from build123d import *

# Parameters (mm, degrees)
SKETCH1_W           = 19.05
SKETCH1_H           = 25.4
BOSS_EXTRUDE1_DEPTH = 6.35
SKETCH2_W           = 6.35
SKETCH2_H           = 6.35
CUT_EXTRUDE1_DEPTH  = 7.35
SKETCH3_W           = 6.35
SKETCH3_H           = 6.35
CUT_EXTRUDE2_DEPTH  = 7.35
SKETCH4_R           = 0.635
CUT_EXTRUDE3_DEPTH  = 7.35
SKETCH5_R           = 0.635
CUT_EXTRUDE4_DEPTH  = 7.35


with BuildPart() as part:
    # Sketch1 → Boss-Extrude1 (new body)
    with BuildSketch(Plane.XY):
        with Locations((9.525, 12.7)):
            Rectangle(SKETCH1_W, SKETCH1_H)
    extrude(amount=BOSS_EXTRUDE1_DEPTH)

    # Sketch2 → Cut-Extrude1 (cut, through all)
    with BuildSketch(Plane(origin=(0, 0, 0), x_dir=(-1, 0, 0), z_dir=(0, 0, -1))):
        with Locations((-3.175, 22.225)):
            Rectangle(SKETCH2_W, SKETCH2_H)
    extrude(amount=-CUT_EXTRUDE1_DEPTH, mode=Mode.SUBTRACT)

    # Sketch3 → Cut-Extrude2 (cut, through all)
    with BuildSketch(Plane(origin=(0, 0, 0), x_dir=(-1, 0, 0), z_dir=(0, 0, -1))):
        with Locations((-15.875, 22.225)):
            Rectangle(SKETCH3_W, SKETCH3_H)
    extrude(amount=-CUT_EXTRUDE2_DEPTH, mode=Mode.SUBTRACT)

    # Sketch4 → Cut-Extrude3 (cut, through all)
    with BuildSketch(Plane(origin=(0, 0, 0), x_dir=(-1, 0, 0), z_dir=(0, 0, -1))):
        with Locations((-9.525, 22.225)):
            Circle(SKETCH4_R)
    extrude(amount=-CUT_EXTRUDE3_DEPTH, mode=Mode.SUBTRACT)

    # Sketch5 → Cut-Extrude4 (cut, through all)
    with BuildSketch(Plane.XY.offset(6.35)):
        with Locations((14.2875, 3.922050028)):
            Circle(SKETCH5_R)
        with Locations((9.525, 3.922050028)):
            Circle(SKETCH5_R)
        with Locations((4.7625, 3.922050028)):
            Circle(SKETCH5_R)
    extrude(amount=-CUT_EXTRUDE4_DEPTH, mode=Mode.SUBTRACT)


solid = part.part
Source: CAD feature listing. Evaluate the final solid. Frame: model axes, mm. A direction names the side the tool comes from. Round coordinates to 2 decimals unless told otherwise and drop trailing zeros. Order: outer loops, then holes, each group sorted by start corner. A loop starts at its lowest first (then second) coordinate and runs counter-clockwise, first axis right, second up. Notation, with made-up numbers: (65.25, 45.25) - (91.25, 45.25) arc R27 cw to (91.25, 69.25) - close; hole circle Ø4 at (34.5, -27.75). An arc over 180 degrees is marked (long way). Use a Markdown table: item, result. Add a question column.
1. Section query B-B (z = 3.75). Give the number of separate pieces and of enclosed holes in the cut face, then the cut area to 3 significant figures.
2. Mould query, pull axis Y, two halves, no side actions, for faces 4 (the flat face through (12.7, 22, 3)), 5 (the cylindrical face through (9.608, 22.855, 3.131)), 6 (the flat face through (9, 0, 3)), 7 (the flat face through (9, 25.4, 3)). Classes: +Y half, -Y half, draft (parallel to the pull), parting line (faces both ways), or undercut.
3. Section query D-D (x = 2.75). Return the cut outline in (y, z), then the cut area to 3 significant figures.
4. Set-up query: faces 1 (the flat face through (16, 19.05, 3)), 2 (the flat face through (6.35, 22, 3)), 3 (the cylindrical face through (8.89, 3.95, 3.22)). Return all of +Z, -Z, +X, -X, +Y, -Y with unobstructed straight access to the full face (end or side cutting, diameter ignored); none if empty.
5. Section query A-A (x = 9.25). Return the cut outline in (y, z), then the cut area to 3 significant figures.
6. Section query C-C (y = 20.25). Return the cut outline in (x, z).
7. Line query: probe 1 along X at (y, z) = (4, 4.25); probe 2 along Y at (x, z) = (14.25, 2.25); probe 3 along X at (y, z) = (20.25, 4.5). Output: solid intervals per line, ascending.
8. First-contact query: pin 1 (1.1 mm diameter, centred on x = 9.525, y = 22.225, fed in from +Z); pin 2 (3 mm diameter, centred on y = 21, z = 3, fed in from -X); pin 3 (3 mm diameter, centred on x = 15.5, z = 1.5, fed in from +Y). Flat tips, straight axial feed; report the tip coordinate or a pass-through.
Derived:
| question | item | result |
|---|---|---|
| 1 | separate pieces | 1 |
| 1 | enclosed holes | 4 |
| 1 | area | 398 mm2 |
| 2 | face 4 | draft |
| 2 | face 5 | undercut |
| 2 | face 6 | -Y half |
| 2 | face 7 | +Y half |
| 3 | outline | (0, 0) - (19.05, 0) - (19.05, 6.35) - (0, 6.35) - close |
| 3 | area | 121 mm2 |
| 4 | face 1 | +Z, -Z, +X, +Y |
| 4 | face 2 | +Z, -Z, -X, +Y |
| 4 | face 3 | +Z, -Z |
| 5 | outline | (0, 0) - (3.35, 0) - (3.35, 6.35) - (0, 6.35) - close; (4.49, 0) - (21.65, 0) - (21.65, 6.35) - (4.49, 6.35) - close; (22.8, 0) - (25.4, 0) - (25.4, 6.35) - (22.8, 6.35) - close |
| 5 | area | 147 mm2 |
| 6 | outline | (6.35, 0) - (12.7, 0) - (12.7, 6.35) - (6.35, 6.35) - close |
| 7 | probe 1 | 0 to 4.13, 5.39 to 8.89, 10.16 to 13.66, 14.92 to 19.05 |
| 7 | probe 2 | 0 to 3.29, 4.56 to 19.05 |
| 7 | probe 3 | 6.35 to 12.7 |
| 8 | pin 1 | through |
| 8 | pin 2 | x = 6.35 |
| 8 | pin 3 | y = 19.05 |
